Here's how the part is built. I have some questions about the finished solid (model axes, mm). A direction names the side the tool comes from. Coordinates: 2 decimals unless noted, no trailing zeros. Write each loop counter-clockwise with the first axis right and the second up, starting at its lowest first coordinate (ties: lowest second). Pieces come first, ordered by that corner, then holes. Notation, with made-up numbers: (42, 7) -> (69, 7) arc R31 ccw to (69, 33) -> close; hole circle Ø6 at (57.5, -15). An arc over 180 degrees is marked (long way). Put each result on its own line as item: value.
Autodesk Inventor part; units mm, degrees
ref_plane "YZ Plane" through (0, 0, 0) normal (1, 0, 0) x (0, 1, 0)
ref_plane "XZ Plane" through (0, 0, 0) normal (0, 1, 0) x (-1, 0, 0)
ref_plane "XY Plane" through (0, 0, 0) normal (0, 0, 1) x (1, 0, 0)
sketch "Sketch1" plane through (0, 0, 0) normal (0, 0, 1) x (1, 0, 0)
  line L0 (40, 21) -> (41, 20)
  line L1 (40, 21) -> (32, 21)
  line L2 (32, 21) -> (32, 16)
  line L3 (32, 16) -> (35, 16)
  arc A0 (36, 15) -> (35, 16) centre (35, 15) ccw
  line L4 (36, 15) -> (36, 8)
  arc A1 (32, 4) -> (36, 8) centre (32, 8) ccw
  line L5 (32, 4) -> (15, 4)
  arc A2 (11.4706, 6.1176) -> (15, 4) centre (15, 8) ccw
  arc A3 (11.4706, 6.1176) -> (11.4706, -6.1176) centre (0, 0) ccw
  arc A4 (15, -4) -> (11.4706, -6.1176) centre (15, -8) ccw
  line L6 (15, -4) -> (32, -4)
  arc A5 (36, -8) -> (32, -4) centre (32, -8) ccw
  line L7 (36, -8) -> (36, -20.0526)
  line L8 (36, -20.0526) -> (39.035, -20.6277)
  line L9 (41, -19) -> (39.035, -20.6277)
  line L10 (41, -19) -> (41, 20)
  circle A6 centre (17, 0) radius 1.5
  circle A7 centre (32, 0) radius 1.5
  circle A8 centre (0, 0) radius 8.65
  line L11 (32, 0) -> (17, 0)
  line L12 (32, 0) -> (17, 0) construction
  line L13 (32, 4) -> (17, 4)
  line L14 (17, -4) -> (32, -4)
  arc A9 (32, -4) -> (32, 4) centre (32, 0) ccw
  arc A10 (17, 4) -> (17, -4) centre (17, 0) ccw
  point P0 (0, 0)
  point P1 (24.5, 0)
  dimension "d0" = 7.5
  dimension "d1" = 8
extrude "Extrusion1" add sketch "Sketch1" along normal blind 3.5 contours L6 A10 L5 A9
thicken "Thicken1" operation add thickness 1.5 both sides no extend neighbours yes toward (0, 0, 1) faces at (22.4427, 2.899, 3.5)
sketch "Sketch2" plane through (17, 4, 5) normal (0, 0, 1) x (1, 0, 0)
  circle A0 centre (8.2825, 2.7175) radius 1.175
  circle A1 centre (8.2825, 2.7175) radius 2.7175
  line L0 (15, 0) -> (0, 0)
  line L1 (11, 2.7175) -> (8.2825, 2.7175)
  line L2 (8.2825, 2.7175) -> (5.565, 2.7175)
  line L3 (5.565, 2.7175) -> (5.565, 0)
  line L4 (11, 2.7175) -> (11, 0)
  point P0 (-17, -4)
extrude "Extrusion2" add sketch "Sketch2" against normal blind 3.5 contours L1 A1 L2 A0 | A0 L2 A1 L1 | L4 L0 A1 | A1 L0 L3
fillet "Fillet1" radius 2 3 edges at (25.2825, 4, 1.5) (22.565, 4, 3.25) (28, 4, 3.25)
properties part number "switch_holder"
Item 1: Imagine slicing it at C-C on x = 31.25. Write out the boundary of the cut face in (y, z), then the cut area to 3 significant figures.
Output:
outline: (-4, 0) -> (-1.3, 0) -> (-1.3, 5) -> (-4, 5) -> close; (1.3, 0) -> (4, 0) -> (4, 5) -> (1.3, 5) -> close
area: 27.0 mm²
Item 2: If we mould it in two halves opening along X, with no side actions, what happens to faces 4 (the cylindrical face through (30.5, -0.07, 2.46)), 5 (the cylindrical face through (21.964, 4.57, 3.091)), 6 (the flat face through (31, 4, 2))? For each: released by +X, released by -X, zero draft, split by the parting line, or undercut.
Output:
face 4: undercut
face 5: released by -X
face 6: zero draft
Item 3: Please list where these lines run through material, in increasing order: line 1 along X through (y, z) = (-1, 2.5); line 2 along Y through (x, z) = (17, 3.1); line 3 along X through (y, z) = (0.75, 4.45). Write a range as from..to.
Output:
line 1: x = 13.13..15.88, 18.12..30.88, 33.12..35.87
line 2: y = -4..-1.5, 1.5..4
line 3: x = 13.07..15.7, 18.3..30.7, 33.3..35.93
Item 4: Which directions (+Z, -Z, +X, -X, +Y, -Y) give clear straight access to the entire face, cutting with the end or side of a thin tool? Please do faces 1 (the cylindrical face through (25.825, 5.675, 3.255)), 2 (the flat face through (25.3, 8.1, 1.5)), 3 (the flat face through (19, 4, 2)).
Output:
face 1: +Z, -Z
face 2: -Z, +X, -X, +Y
face 3: +Z, -Z, -X, +Y
Item 5: For P1, Ø2.5, axis at x = 32, y = 0, coming from the +Z side; P2, Ø4, axis at x = 25.28, y = 6.72, coming from the +Z side; P3, Ø1.5, axis at y = -1, z = 4.5, coming from the -X side; P4, Ø1, axis at x = 26.5, y = 8, coming from the -Z side, each with a flat end and sliding along its axis, tell me the tip position at first contact or that it passes through.
Output:
P1: passes through
P2: stops at z = 5
P3: stops at x = 13.01
P4: stops at z = 1.5
Item 6: Imagine slicing it at D-D on y = 7. Write out the boundary of the cut face in (x, z).
Output:
outline: (22.58, 1.5) -> (24.14, 1.5) -> (24.14, 5) -> (22.58, 5) -> close; (26.42, 1.5) -> (27.99, 1.5) -> (27.99, 5) -> (26.42, 5) -> close
Item 7: Imagine slicing it at A-A on z = 2.05. State how many separate pieces and enclosed holes the cut face has, then the cut area to 3 significant figures.
Output:
separate pieces: 1
enclosed holes: 3
area: 180 mm²
Item 8: Imagine slicing it at B-B on y = 0. Write out the boundary of the cut face in (x, z).
Output:
outline: (13, 0) -> (15.5, 0) -> (15.5, 5) -> (13, 5) -> close; (18.5, 0) -> (30.5, 0) -> (30.5, 5) -> (18.5, 5) -> close; (33.5, 0) -> (36, 0) -> (36, 5) -> (33.5, 5) -> close
